Geometry check sheet. Reference: drawing and pictorial views, mm from the part's lowest x, y, z. Coordinates: 2 decimals unless noted, no trailing zeros. Loops run counter-clockwise (first coordinate to the right, second up) from the corner with the lowest first, then second, coordinate; pieces in that order, holes last. Notation, with made-up numbers: (-2, 13) -> (57, 13) arc R30 ccw to (57, 52) -> close; hole circle Ø10 at (51, 25.25). An arc over 180 degrees is marked (long way). Use one line per item in the form item = value.
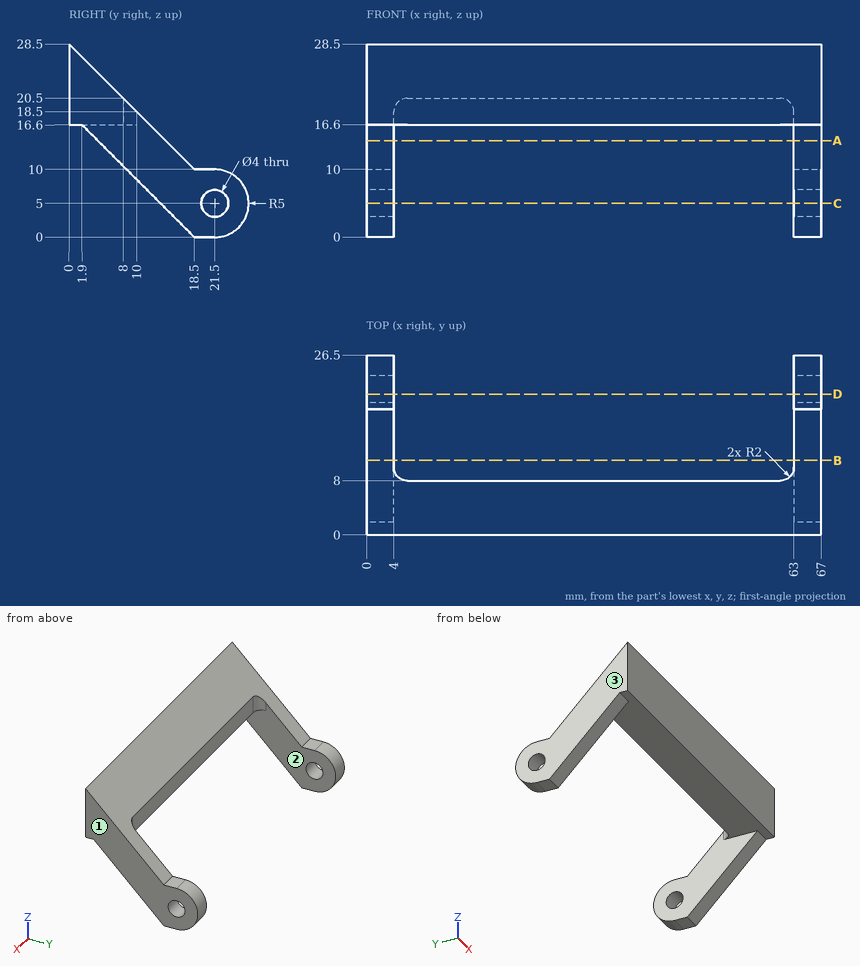
(1) Section check A-A, the plane z = 14.25. Record the boundary of the cut face in (x, y).
Established:
outline = (0, 4.25) -> (4, 4.25) -> (4, 14.25) -> (0, 14.25) -> close; (63, 4.25) -> (67, 4.25) -> (67, 14.25) -> (63, 14.25) -> close
(2) Mould release check, pull along X, two halves, no side actions. Record for the marked faces 1, 2 and 3: +X half, -X half, draft (parallel to the pull), parting line (faces both ways), or undercut.
Established:
face_1 = +X half
face_2 = undercut
face_3 = -X half
(3) Section check C-C, the plane z = 5. Record the boundary of the cut face in (x, y).
Established:
outline = (0, 13.5) -> (4, 13.5) -> (4, 19.5) -> (0, 19.5) -> close; (0, 23.5) -> (4, 23.5) -> (4, 26.5) -> (0, 26.5) -> close; (63, 13.5) -> (67, 13.5) -> (67, 19.5) -> (63, 19.5) -> close; (63, 23.5) -> (67, 23.5) -> (67, 26.5) -> (63, 26.5) -> close
(4) Section check B-B, the plane y = 11. Record the boundary of the cut face in (x, z), plus the area to 3 significant figures.
Established:
outline = (0, 7.5) -> (4, 7.5) -> (4, 17.5) -> (0, 17.5) -> close; (63, 7.5) -> (67, 7.5) -> (67, 17.5) -> (63, 17.5) -> close
area = 80.0 mm²
(5) Go/stop test with flat-tipped pins: P1, Ø2.5, axis at x = 65, y = 20, coming from the +Z side; P2, Ø3, axis at x = 23, z = 18.5, coming from the +Y side; P3, Ø3, axis at x = 31.5, y = 5.5, coming from the -Z side. Record where each tip stops, or that it passes through.
Established:
P1 = 10
P2 = 8
P3 = 16.6
(6) Scan lines: line 1 along X through (y, z) = (10, 8.75); line 2 along Y through (x, z) = (65.8, 5); line 3 along Z through (x, y) = (63.5, 6.75). Record each from-to range of solid material in increasing order.
Established:
line_1 = 0 to 4, 63 to 67
line_2 = 13.5 to 19.5, 23.5 to 26.5
line_3 = 11.75 to 21.75
(7) Section check D-D, the plane y = 20.75. Record the boundary of the cut face in (x, z), plus the area to 3 significant figures.
Established:
outline = (0, 0) -> (4, 0) -> (4, 3.15) -> (0, 3.15) -> close; (0, 6.85) -> (4, 6.85) -> (4, 10) -> (0, 10) -> close; (63, 0) -> (67, 0) -> (67, 3.15) -> (63, 3.15) -> close; (63, 6.85) -> (67, 6.85) -> (67, 10) -> (63, 10) -> close
area = 50.3 mm²
